The model under review builds one solid part; all positions refer to its coordinate system, in mm. A direction names the side the tool comes from. Give positions to 0.01 mm unless a question says otherwise; leave off trailing zeros. Loops run counter-clockwise (first coordinate to the right, second up) from the corner with the lowest first, then second, coordinate; pieces in that order, holes last. Notation, with made-up numbers: (4, -8) - (48, -8) arc R16 cw to (48, 10) - close; hole circle Ø5 at (55, -34). An arc over 180 degrees is marked (long way). Answer as a JSON object with one key per item and string values.
from build123d import *

# Parameters (mm, degrees)
EXTRUDE_THIN1_DEPTH       = 80
BOSS_EXTRUDE1_START       = -10
BOSS_EXTRUDE1_DEPTH       = 10
SKETCH3_R                 = 2.25
BOSS_EXTRUDE2_DEPTH       = 5
BOSS_EXTRUDE3_DEPTH       = 10
SKETCH5_R                 = 2.25
CUT_EXTRUDE1_DEPTH        = 6
BOSS_EXTRUDE4_REACH       = 104.415
BOSS_EXTRUDE4_END_RADIUS  = 39
SKETCH10_W                = 20
SKETCH10_H                = 20
BOSS_EXTRUDE6_DEPTH       = 6
BOSS_EXTRUDE7_START       = -38.548677333
BOSS_EXTRUDE7_OUTLINE_W   = 20
BOSS_EXTRUDE7_OUTLINE_H   = 20
BOSS_EXTRUDE7_DEPTH       = 38.548677333
BOSS_EXTRUDE7_START_2     = 88.145703723
BOSS_EXTRUDE7_2_OUTLINE_W = 23
BOSS_EXTRUDE7_2_OUTLINE_H = 23
BOSS_EXTRUDE7_2_DEPTH     = 1.854296277
BOSS_EXTRUDE9_DEPTH       = 20
SKETCH16_R                = 2.5
CUT_EXTRUDE2_DEPTH        = 20


with BuildPart() as part:
    # Sketch1 → Extrude-Thin1 (new body)
    with BuildSketch(Plane.XY):
        with BuildLine():
            ThreePointArc((-35, 0), (0, -35), (35, 0))
            Line((35, 0), (39, 0))
            ThreePointArc((39, 0), (0, -39), (-39, 0))
            Line((-39, 0), (-35, 0))
        make_face()
    extrude(amount=EXTRUDE_THIN1_DEPTH)

    # Sketch2 → Boss-Extrude1 (add)
    with BuildSketch(Plane.XY.offset(80).offset(BOSS_EXTRUDE1_START)):
        with BuildLine():
            Line((0, -39), (0, -35))
            Line((0, -35), (-10, -35))
            Line((-10, -35), (-10, -37.69615365))
            ThreePointArc((-10, -37.69615365), (-5.042321274, -38.672664715), (0, -39))
        make_face()
        with BuildLine():
            Line((10, -35), (0, -35))
            Line((0, -35), (0, -39))
            ThreePointArc((0, -39), (5.042321274, -38.672664715), (10, -37.69615365))
            Line((10, -37.69615365), (10, -35))
        make_face()
        with BuildLine():
            ThreePointArc((10, -37.69615365), (5.042321274, -38.672664715), (0, -39))
            ThreePointArc((0, -39), (-5.042321274, -38.672664715), (-10, -37.69615365))
            Line((-10, -37.69615365), (-10, -43))
            Line((-10, -43), (10, -43))
            Line((10, -43), (10, -37.69615365))
        make_face()
    extrude(amount=BOSS_EXTRUDE1_DEPTH)

    # Sketch3 → Boss-Extrude2 (add)
    with BuildSketch(Plane.XY.offset(80)):
        with Locations((-5, -39)):
            Circle(SKETCH3_R)
        with Locations((5, -39)):
            Circle(SKETCH3_R)
    extrude(amount=BOSS_EXTRUDE2_DEPTH)

    # Sketch4 → Boss-Extrude3 (add)
    with BuildSketch(Plane(origin=(0, 0, 0), x_dir=(-1, 0, 0), z_dir=(0, 0, -1))):
        with BuildLine():
            Line((0, -39), (0, -35))
            Line((0, -35), (-10, -35))
            Line((-10, -35), (-10, -37.69615365))
            ThreePointArc((-10, -37.69615365), (-5.042321274, -38.672664715), (0, -39))
        make_face()
        with BuildLine():
            ThreePointArc((10, -37.69615365), (5.042321274, -38.672664715), (0, -39))
            ThreePointArc((0, -39), (-5.042321274, -38.672664715), (-10, -37.69615365))
            Line((-10, -37.69615365), (-10, -43))
            Line((-10, -43), (10, -43))
            Line((10, -43), (10, -37.69615365))
        make_face()
        with BuildLine():
            Line((10, -35), (0, -35))
            Line((0, -35), (0, -39))
            ThreePointArc((0, -39), (5.042321274, -38.672664715), (10, -37.69615365))
            Line((10, -37.69615365), (10, -35))
        make_face()
    extrude(amount=-BOSS_EXTRUDE3_DEPTH)

    # Sketch5 → Cut-Extrude1 (cut)
    with BuildSketch(Plane(origin=(0, 0, 0), x_dir=(-1, 0, 0), z_dir=(0, 0, -1))):
        with Locations(Location((-5, -39, 0), (0, 0, 180))):
            Circle(SKETCH5_R)
        with Locations(Location((5, -39, 0), (0, 0, 180))):
            Circle(SKETCH5_R)
    extrude(amount=-CUT_EXTRUDE1_DEPTH, mode=Mode.SUBTRACT)

    # Boss-Extrude4: up to this cylinder (the profile starts outside it)
    boss_extrude4_end = Plane(origin=(0, 0, 40), z_dir=(0, 0, -1)) * Cylinder(BOSS_EXTRUDE4_END_RADIUS, 287.83, mode=Mode.PRIVATE)
    # Sketch10 → Boss-Extrude4 (add, up to the surface)
    with BuildSketch(Plane(origin=(0, -49.619293796, 4.341125699), x_dir=(1, 0, 0), z_dir=(0, 0.9961946980917462, -0.08715574274765152)), mode=Mode.PRIVATE) as boss_extrude4_sk1:
        with Locations((0, -35.795085407)):
            Rectangle(SKETCH10_W, SKETCH10_H)
    boss_extrude4_tool1 = extrude(boss_extrude4_sk1.sketch, amount=BOSS_EXTRUDE4_REACH, mode=Mode.PRIVATE) - boss_extrude4_end
    add(boss_extrude4_tool1.solids().sort_by_distance((0, -46.499547, 40))[0])

    # Sketch14 → Boss-Extrude6 (add)
    with BuildSketch(Plane(origin=(0, -0.732594735, -5.56460947), x_dir=(1, 0, 0), z_dir=(0, 0.130526192220045, 0.9914448613738114))):
        with BuildLine():
            Line((-39, 0), (-39, 50))
            Line((-39, 50), (39, 50))
            Line((39, 50), (39, 0))
            ThreePointArc((39, 0), (0, -39), (-39, 0))
        make_face()
    extrude(amount=BOSS_EXTRUDE6_DEPTH)

    # Boss-Extrude7: read off the stored shape, not the designer's step
    # Boss-Extrude7 outline → Boss-Extrude7 (add)
    with BuildSketch(Plane(origin=(0, -49.619293796, 4.341125699), x_dir=(1, 0, 0), z_dir=(0, 0.9961946980917462, -0.08715574274765152)).offset(BOSS_EXTRUDE7_START)):
        with Locations((0, -35.795085407)):
            Rectangle(BOSS_EXTRUDE7_OUTLINE_W, BOSS_EXTRUDE7_OUTLINE_H)
    extrude(amount=BOSS_EXTRUDE7_DEPTH)

    # Boss-Extrude7 2 outline → Boss-Extrude7 2 (cut)
    with BuildSketch(Plane(origin=(0, 0, 0), x_dir=(0.9994119135527714, 0.03413748045727771, -0.003234111441613329), z_dir=(0.0342903346263607, -0.9949568891477218, 0.09426007473315608)).offset(BOSS_EXTRUDE7_START_2)):
        with Locations((-3.5, 35.5)):
            Rectangle(BOSS_EXTRUDE7_2_OUTLINE_W, BOSS_EXTRUDE7_2_OUTLINE_H)
    extrude(amount=BOSS_EXTRUDE7_2_DEPTH, mode=Mode.SUBTRACT)

    # Sketch15 → Boss-Extrude9 (add, along a direction that is not the sketch's normal)
    with BuildSketch(Plane(origin=(10, 0, 0), x_dir=(0, 0, -1), z_dir=(1, 0, 0))):
        Polygon((-53.249344589, -83.203115712), (-33.337982915, -85.089475272), (-32.46309628, -75.089475272), (-52.374457954, -73.203115712), align=None)
    extrude(amount=BOSS_EXTRUDE9_DEPTH, dir=(0.9994118831812419, 0.034160731366783506, -0.0029886767323038838))

    # Sketch16 → Cut-Extrude2 (cut)
    with BuildSketch(Plane(origin=(2.678543813, -77.719732066, 7.363000179), x_dir=(0.9994101830326216, 0.03396190638807467, -0.005086744065644862), z_dir=(-0.03429033462636075, 0.9949568891477218, -0.0942600747331567))):
        with Locations(Location((17.250851161, -40.271437351, 0), (0, 0, 269.893376297))):
            Circle(SKETCH16_R)
        with Locations(Location((17.269461459, -30.270938076, 0), (0, 0, 269.893376297))):
            Circle(SKETCH16_R)
    extrude(amount=-CUT_EXTRUDE2_DEPTH, mode=Mode.SUBTRACT)


solid = part.part
Q1. For faces 4 (the face through (-39, 24, -6)), 5 (the face through (5, -39, 6)), 6 (the face through (0, -43, 5)), 7 (the face through (-37, 0, 39)), 8 (the face through (-0.77, -34.99, 39.64)), list the 3-axis set-ups (+Z, -Z, +X, -X, +Y, -Y) from which the entire face can be reached by the end or side of a thin tool; tool diameter is ignored.
Results:
{"face 4": "+Z, -Z, -X, +Y, -Y", "face 5": "none", "face 6": "-Z, +X, -X, -Y", "face 7": "+Z, +X, -X, +Y", "face 8": "+Z, +Y"}
Q2. To check wall thickness, follow probe 1 along X at (y, z) = (-39, 3); probe 2 along X at (y, z) = (-2, 40.5); probe 3 along Y at (x, z) = (16.5, 50). State the ranges of each line that lie inside material, in increasing order. Write a range as [from, to].
Results:
{"probe 1": "x = [-10, -7.25], [-2.75, 2.75], [7.25, 10]", "probe 2": "x = [-38.95, -34.94], [34.94, 38.95]", "probe 3": "y = [-83.29, -73.2], [-35.34, -30.87]"}
Q3. Consider section B-B, the plane x = 0. State the section outline as (y, z) points.
Results:
{"outline": "(-85.43, 33.37) - (-39, 29.31) - (-39, 10) - (-43, 10) - (-43, 0) - (-39.34, 0) - (-39.4, -0.47) - (48.84, -12.09) - (49.62, -6.14) - (-35, 5) - (-35, 80) - (-43, 80) - (-43, 70) - (-39, 70) - (-39, 49.38) - (-83.54, 53.28) - close"}
Q4. Consider section D-D, the plane z = 21.5. State the section outline as (x, y) points.
Results:
{"outline": "(-39, 0) arc R39 ccw to (39, 0) - (35, 0) arc R35 cw to (-35, 0) - close"}
Q5. Consider section A-A, the plane z = 77.5. State the section outline as (x, y) points.
Results:
{"outline": "(-39, 0) arc R39 ccw to (-10, -37.7) - (-10, -43) - (10, -43) - (10, -37.7) arc R39 ccw to (39, 0) - (35, 0) arc R35 cw to (-35, 0) - close"}
Q6. The part is to be moulded in two halves that separate along X. For faces 1 (the face through (-10, -61, 41)), 2 (the face through (0.55, 7.9, -0.65)), 3 (the face through (10, -40, 75)), say which applies: +X half, -X half, draft (parallel to the pull), parting line (faces both ways), or undercut.
Results:
{"face 1": "-X half", "face 2": "undercut", "face 3": "+X half"}
Q7. Consider section C-C, the plane y = 12.5. State the section outline as (x, z) points.
Results:
{"outline": "(-39, -7.31) - (39, -7.31) - (39, -1.25) - (-39, -1.25) - close"}
Q8. Clearance check with flat-ended pins moving along their axes: pin 1 Ø1.6 at (y, z) = (-41, 75.5) entering from -X; pin 2 Ø1.6 at (y, z) = (-41, 6) entering from +X; pin 3 Ø13 at (y, z) = (-76.5, 40) entering from +X. State where each tip first meets the part, or that it passes through.
Results:
{"pin 1": "stops at x = -10", "pin 2": "stops at x = 10", "pin 3": "stops at x = 29.99"}
